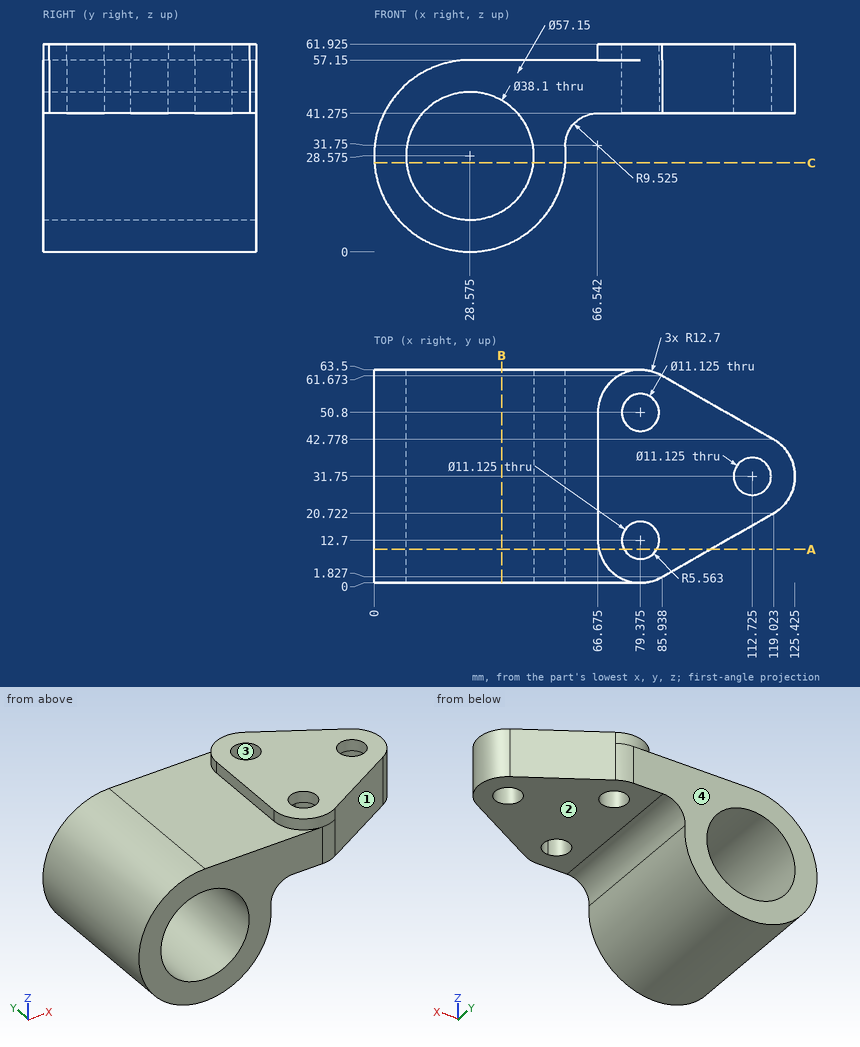
Geometry: see drawing. Coordinates: mm, zero at the bounding-box minimum. Coordinates: 2 decimals unless noted, no trailing zeros. Loops run counter-clockwise (first coordinate to the right, second up) from the corner with the lowest first, then second, coordinate; pieces in that order, holes last. Notation, with made-up numbers: M 4.25,45.25 L 48.25,45.25 A18 cw 48.25,75.25 Z; hole C -9,37 d7. An arc over 180 degrees is marked long. Answer in a Markdown table with one row per item.
Q1. Section C-C on z = 26.5. Return the cut outline in (x, y) (1 decimal), plus the area to 3 significant figures.
Answers below:
| item | result |
|---|---|
| outline | M 0.1,0 L 9.6,0 L 9.6,63.5 L 0.1,63.5 Z; M 47.5,0 L 57.1,0 L 57.1,63.5 L 47.5,63.5 Z |
| area | 1,210 mm^2 |
Q2. First-contact query: pin 1 (2 mm diameter, centred on x = 14.5, y = 14, fed in from +Z); pin 2 (10 mm diameter, centred on x = 99.5, z = 54.5, fed in from +Y); pin 3 (13 mm diameter, centred on x = 112.73, y = 31.75, fed in from +Z) (1 decimal); pin 4 (9 mm diameter, centred on x = 79.375, y = 12.7, fed in from +Z). Flat tips, straight axial feed; report the tip coordinate or a pass-through.
Answers below:
| item | result |
|---|---|
| pin 1 | stops at z = 53.98 |
| pin 2 | stops at y = 56.78 |
| pin 3 | stops at z = 61.9 |
| pin 4 | passes through |
Q3. Ray query, probe 1 along Z at (x, y) = (94.5, 7.5) (1 decimal); probe 2 along Z at (x, y) = (42, 4); probe 3 along Z at (x, y) = (29, 37.5). Return the intervals inside material, ascending. Write a range as from..to.
Answers below:
| item | result |
|---|---|
| probe 1 | z = 41.3..61.9 |
| probe 2 | z = 3.35..15.06, 42.09..57.15 |
| probe 3 | z = 0..9.53, 47.62..57.15 |
Q4. Section B-B on x = 38. Return the cut outline in (y, z), plus the area to 4 significant figures.
Answers below:
| item | result |
|---|---|
| outline | M 0,1.6 L 63.5,1.6 L 63.5,12.02 L 0,12.02 Z; M 0,45.13 L 63.5,45.13 L 63.5,57.15 L 0,57.15 Z |
| area | 1,425 mm^2 |
Q5. Draft query along Y for the marked faces 1, 2, 3 and 4. Return one class per face: pulls with the +Y half, pulls with the -Y half, needs draft (parallel to the pull), parting line crosses it, or undercut.
Answers below:
| item | result |
|---|---|
| face 1 | pulls with the -Y half |
| face 2 | needs draft |
| face 3 | undercut |
| face 4 | pulls with the +Y half |
Q6. Section A-A on y = 10. State how many separate pieces and enclosed holes the cut face has, plus the area to 3 significant figures.
Answers below:
| item | result |
|---|---|
| separate pieces | 2 |
| enclosed holes | 1 |
| area | 2,260 mm^2 |
